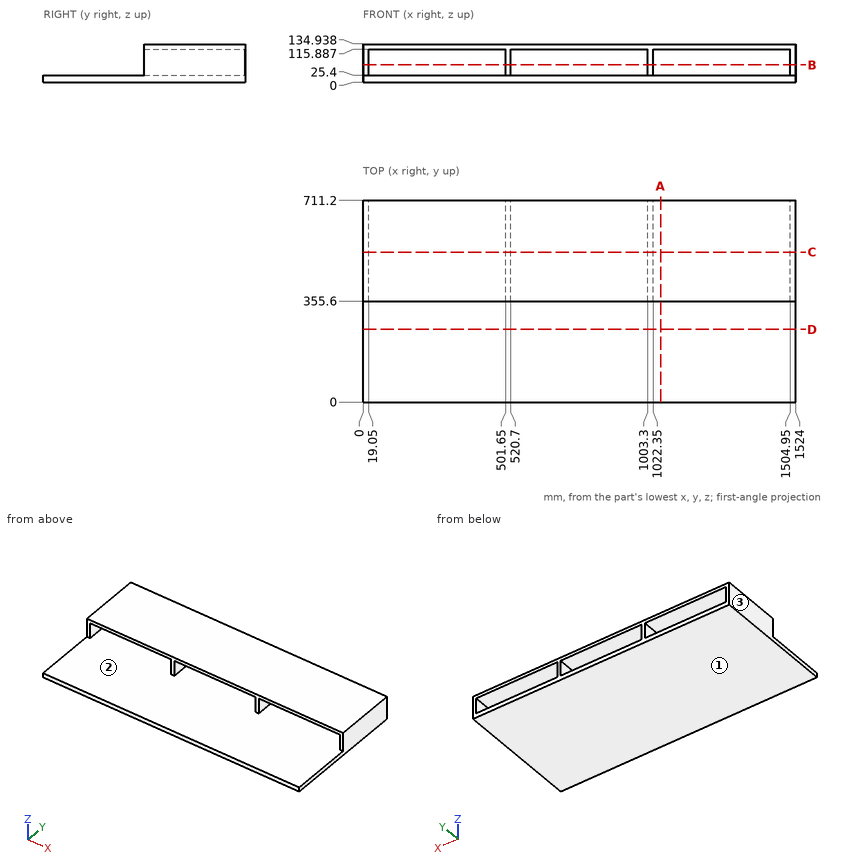
Geometry check sheet. Reference: drawing and pictorial views, mm from the part's lowest x, y, z. Round coordinates to 2 decimals unless told otherwise and drop trailing zeros. Write each loop counter-clockwise with the first axis right and the second up, starting at its lowest first coordinate (ties: lowest second). Pieces come first, ordered by that corner, then holes.
1. Draft check along Z on the marked faces 1, 2 and 3. Enter one of: +Z half, -Z half, draft (parallel to the pull), parting line (faces both ways), or undercut.
2. Section check B-B on z = 61. Enter the section's corners in (x, y), plus the area to 3 significant figures.
3. Section check D-D on y = 256. Enter the section's corners in (x, z), plus the area to 3 significant figures.
4. Scan lines: L1, parallel to X at y = 363, z = 92.5; L2, parallel to Z at x = 200, y = 359.5; L3, parallel to Z at x = 477.5, y = 40.5. Record each from-to range of solid material in increasing order.
5. Section check C-C on y = 528.5. Enter the section's corners in (x, z).
6. Section check A-A on x = 1048.5. Enter the section's corners in (y, z), plus the area to 3 significant figures.
Answer:
1. face 1: -Z half
1. face 2: undercut
1. face 3: draft
2. outline: (0, 355.6) - (19.05, 355.6) - (19.05, 711.2) - (0, 711.2) - close; (501.65, 355.6) - (520.7, 355.6) - (520.7, 711.2) - (501.65, 711.2) - close; (1003.3, 355.6) - (1022.35, 355.6) - (1022.35, 711.2) - (1003.3, 711.2) - close; (1504.95, 355.6) - (1524, 355.6) - (1524, 711.2) - (1504.95, 711.2) - close
2. area: 27,100 mm2
3. outline: (0, 0) - (1524, 0) - (1524, 25.4) - (0, 25.4) - close
3. area: 38,700 mm2
4. L1: x = 0 to 19.05, 501.65 to 520.7, 1003.3 to 1022.35, 1504.95 to 1524
4. L2: z = 0 to 25.4, 115.89 to 134.94
4. L3: z = 0 to 25.4
5. outline: (0, 0) - (1524, 0) - (1524, 134.94) - (0, 134.94) - close; hole (19.05, 25.4) - (501.65, 25.4) - (501.65, 115.89) - (19.05, 115.89) - close; hole (520.7, 25.4) - (1003.3, 25.4) - (1003.3, 115.89) - (520.7, 115.89) - close; hole (1022.35, 25.4) - (1504.95, 25.4) - (1504.95, 115.89) - (1022.35, 115.89) - close
6. outline: (0, 0) - (711.2, 0) - (711.2, 25.4) - (0, 25.4) - close; (355.6, 115.89) - (711.2, 115.89) - (711.2, 134.94) - (355.6, 134.94) - close
6. area: 24,800 mm2
